Read the model definition and answer for the solid it produces. Units are mm, in the model's axes. Face numbers are marked on the shaded views. A direction names the side the tool comes from. Give positions to 0.01 mm unless a question says otherwise; leave off trailing zeros. Write each loop counter-clockwise with the first axis right and the second up, starting at its lowest first coordinate (ties: lowest second). Pieces come first, ordered by that corner, then holes. Notation, with made-up numbers: M 35.25,12 L 42.25,12 A6 ccw 42.25,21 Z; hole C 38.25,3.5 d10. An arc over 180 degrees is marked long. Use a Markdown table: item, result. Add a question column.
Item 1: A cutting plane is placed at B-B on x = 8.5. Determine the outline of the cut face in (y, z), then the cut area to 3 significant figures.
Item 2: Given P1, Ø0.9, axis at x = -10.5, z = 7.5, coming from the +Y side; P2, Ø12, axis at x = 14, y = 36.5, coming from the -Z side; P3, Ø4, axis at x = -12.5, y = 8.5, coming from the +Z side, each flat-ended and moving along its own axis, determine where each tip first touches the part or whether it passes through.
Item 3: For the marked faces 1, 2, 3, 4 and 5, determine the directions among +Z, -Z, +X, -X, +Y, -Y from which every point of the face is accessible in a straight line to the end or side of a thin tool.
Item 4: The mould has two halves that part along Y. Classify the marked faces 6, 7 and 8: pulls with the +Y half, pulls with the -Y half, needs draft (parallel to the pull), parting line crosses it, or undercut.
Item 5: A cutting plane is placed at C-C on z = -13. Determine the outline of the cut face in (x, y), then the cut area to 3 significant figures.
Item 6: A cutting plane is placed at A-A on z = 0. Determine the outline of the cut face in (x, y), then the cut area to 3 significant figures.
Item 7: Consider probe 1 along Y at (x, z) = (0.5, 14); probe 2 along X at (y, z) = (44, 7); probe 3 along X at (y, z) = (43.2, 7.75). Determine where each line is inside the solid, lowest interval first. Write a range as [from, to].
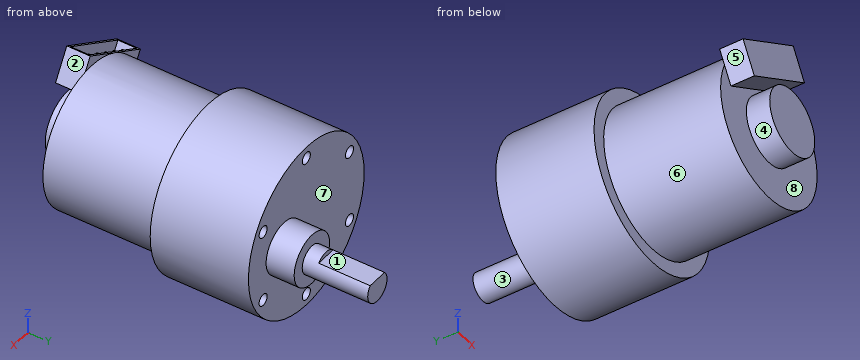
from build123d import *

# Parameters (mm, degrees)
SKETCH_1_R             = 15
EXTRUDE_1_DEPTH        = 25
SKETCH_2_R             = 18
EXTRUDE_2_DEPTH        = 21
SKETCH_3_R             = 5.5
EXTRUDE_3_DEPTH        = 6
SKETCH_4_R             = 3
EXTRUDE_4_DEPTH        = 14
CUT_EXTRUDE_START      = -11
CUT_EXTRUDE_1_DEPTH    = 11
HOLE_WIZARD_M3_1_D     = 2.5
HOLE_WIZARD_M3_1_DEPTH = 5.5
HOLE_WIZARD_M3_1_TIP   = 0.751075774
EXTRUDE_5_DEPTH        = 5
SKETCH_10_R            = 7
EXTRUDE_6_DEPTH        = 5
CUT_EXTRUDE_2_DEPTH    = 6
SKETCH_12_W            = 0.4
SKETCH_12_H            = 0.4
EXTRUDE_7_DEPTH        = 5


with BuildPart() as part:
    # 草图1 → 凸台-拉伸1 (new body)
    with BuildSketch(Plane(origin=(0, 0, 0), x_dir=(1, 0, 0), z_dir=(0, 1, 0))):
        with Locations(Location((0, 0, 0), (0, 0, 270))):
            Circle(SKETCH_1_R)
    extrude(amount=EXTRUDE_1_DEPTH)

    # 草图2 → 凸台-拉伸2 (add)
    with BuildSketch(Plane(origin=(0, 25, 0), x_dir=(1, 0, 0), z_dir=(0, 1, 0))):
        with Locations(Location((0, 0, 0), (0, 0, 90))):
            Circle(SKETCH_2_R)
    extrude(amount=EXTRUDE_2_DEPTH)

    # 草图3 → 凸台-拉伸3 (add)
    with BuildSketch(Plane(origin=(0, 46, 0), x_dir=(1, 0, 0), z_dir=(0, 1, 0))):
        with Locations(Location((7, 0, 0), (0, 0, 270))):
            Circle(SKETCH_3_R)
    extrude(amount=EXTRUDE_3_DEPTH)

    # 草图4 → 凸台-拉伸4 (add)
    with BuildSketch(Plane(origin=(0, 52, 0), x_dir=(1, 0, 0), z_dir=(0, 1, 0))):
        with Locations(Location((7, 0, 0), (0, 0, 270))):
            Circle(SKETCH_4_R)
    extrude(amount=EXTRUDE_4_DEPTH)

    # 草图5 → 切除-拉伸1 (cut)
    with BuildSketch(Plane(origin=(0, 66, 0), x_dir=(1, 0, 0), z_dir=(0, 1, 0)).offset(CUT_EXTRUDE_START)):
        with BuildLine():
            Line((9.236067977, -2), (4.763932023, -2))
            ThreePointArc((4.763932023, -2), (7, -3), (9.236067977, -2))
        make_face()
    extrude(amount=CUT_EXTRUDE_1_DEPTH, mode=Mode.SUBTRACT)

    # M3 螺纹孔1
    with Locations(Plane(origin=(0, 46, 0), x_dir=(1, 0, 0), z_dir=(0, 1, 0))):
        with Locations((0, 15.5), (-13.423393759, 7.75), (-13.423393759, -7.75), (0, -15.5), (13.423393759, -7.75), (13.423393759, 7.75)):
            Hole(HOLE_WIZARD_M3_1_D / 2, depth=HOLE_WIZARD_M3_1_DEPTH)
            with Locations((0, 0, -(HOLE_WIZARD_M3_1_DEPTH + HOLE_WIZARD_M3_1_TIP / 2))):  # 118° drill point
                Cone(0, HOLE_WIZARD_M3_1_D / 2, HOLE_WIZARD_M3_1_TIP, mode=Mode.SUBTRACT)

    # 草图9 → 凸台-拉伸5 (add)
    with BuildSketch(Plane.XZ):
        Polygon((-15.294228634, 8.490381057), (-11.794228634, 2.42820323), (3.794228634, 11.42820323), (0.294228634, 17.490381057), align=None)
    extrude(amount=EXTRUDE_5_DEPTH)

    # 草图10 → 凸台-拉伸6 (add)
    with BuildSketch(Plane.XZ):
        with Locations(Location((0, 0, 0), (0, 0, 90))):
            Circle(SKETCH_10_R)
    extrude(amount=EXTRUDE_6_DEPTH)

    # 草图11 → 切除-拉伸2 (cut)
    with BuildSketch(Plane(origin=(-7.5, 0, 12.990381057), x_dir=(0.8660254037844379, 0, 0.5000000000000013), z_dir=(-0.5000000000000013, 0, 0.8660254037844379))):
        Polygon((8.5, -0.5), (0, -0.5), (-8.5, -0.5), (-8.5, -4.5), (8.5, -4.5), align=None)
    extrude(amount=-CUT_EXTRUDE_2_DEPTH, mode=Mode.SUBTRACT)

    # 草图12 → 凸台-拉伸7 (add)
    with BuildSketch(Plane(origin=(-4.5, 0, 7.794228634), x_dir=(0.8660254037844379, 0, 0.5000000000000013), z_dir=(-0.5000000000000013, 0, 0.8660254037844379))):
        with Locations((-7.5, -2.5)):
            Rectangle(SKETCH_12_W, SKETCH_12_H)
        with Locations((-4.5, -2.5)):
            Rectangle(SKETCH_12_W, SKETCH_12_H)
        with Locations((-1.5, -2.5)):
            Rectangle(SKETCH_12_W, SKETCH_12_H)
        with Locations((1.5, -2.5)):
            Rectangle(SKETCH_12_W, SKETCH_12_H)
        with Locations((4.5, -2.5)):
            Rectangle(SKETCH_12_W, SKETCH_12_H)
        with Locations((7.5, -2.5)):
            Rectangle(SKETCH_12_W, SKETCH_12_H)
    extrude(amount=EXTRUDE_7_DEPTH)


solid = part.part
Filled in:
| question | item | result |
|---|---|---|
| 1 | outline | M 0,-12.36 L 25,-12.36 L 25,-15.87 L 46,-15.87 L 46,-5.29 L 52,-5.29 L 52,-2.6 L 66,-2.6 L 66,2 L 55,2 L 55,2.6 L 52,2.6 L 52,5.29 L 46,5.29 L 46,15.87 L 25,15.87 L 25,12.36 L 0,12.36 Z |
| 1 | area | 1,410 mm² |
| 2 | P1 | y = 46 |
| 2 | P2 | z = -16.12 |
| 2 | P3 | z = 10.71 |
| 3 | face 1 | +Z, +X, -X, +Y |
| 3 | face 2 | +Z, +X, -Y |
| 3 | face 3 | +Y |
| 3 | face 4 | -Y |
| 3 | face 5 | -Z, -X, -Y |
| 4 | face 6 | undercut |
| 4 | face 7 | pulls with the +Y half |
| 4 | face 8 | pulls with the -Y half |
| 5 | outline | M -12.45,25 L -7.48,25 L -7.48,0 L 7.48,0 L 7.48,25 L 12.45,25 L 12.45,46 L -12.45,46 Z |
| 5 | area | 897 mm² |
| 6 | outline | M -18,25 L -15,25 L -15,0 L -7,0 L -7,-5 L 7,-5 L 7,0 L 15,0 L 15,25 L 18,25 L 18,46 L 12.5,46 L 12.5,52 L 10,52 L 10,66 L 4,66 L 4,52 L 1.5,52 L 1.5,46 L -18,46 Z |
| 6 | area | 1,730 mm² |
| 7 | probe 1 | [-5, -4.5], [-2.7, -2.3], [-0.5, 46] |
| 7 | probe 2 | [-16.58, -14.42], [-12.42, 12.42], [14.42, 16.58] |
| 7 | probe 3 | [-16.25, -14.67], [-12.17, 12.17], [14.67, 16.25] |
